Input: part model. Units: mm. Frame: model coordinates. A direction names the side the tool comes from. Round coordinates to 2 decimals unless told otherwise and drop trailing zeros. Loops run counter-clockwise (first coordinate to the right, second up) from the corner with the lowest first, then second, coordinate; pieces in that order, holes last.
(1) Cut plane C-C, the plane z = 80. Output: boundary loops of the cut face in (x, y).
(2) Draft query along Z for faces 3 (the face through (-29, 11, 111.427)), 4 (the face through (-84.149, 12, -41)), 5 (the face through (-27, 11, -194.573)). Return one class per face: released by +Z, released by -Z, zero draft, split by the parting line, or undercut.
(3) Line query: line 1 (X direction, y = 18, z = -43.75); line 2 (X direction, y = 10.75, z = -59.5); line 3 (Z direction, x = -60.5, y = 21.75). Output: solid intervals per line, ascending.
(4) Cut plane B-B, the plane x = -9. Output: boundary loops of the cut face in (y, z), and give its area (3 significant figures).
(5) First-contact query: pin 1 Ø5 at (x, z) = (-52, -162.5) entering from +Y. Flat tip, straight axial feed; report the tip coordinate or a pass-through.
(6) Access query for faces 1 (the face through (-27, -1, -39)), 2 (the face through (-29, 11, 109.927)). Directions: +Z, -Z, +X, -X, +Y, -Y. A direction counts if a zero-diameter tool reaches every point of the face in a straight line with its end or side. Return the directions, or none.
(7) Cut plane A-A, the plane y = 10.25. Output: boundary loops of the cut face in (x, z), and give its area (3 significant figures).
Autodesk Inventor part; units mm, degrees
ref_plane "YZ Plane" through (0, 0, 0) normal (1, 0, 0) x (0, 1, 0)
ref_plane "XZ Plane" through (0, 0, 0) normal (0, 1, 0) x (-1, 0, 0)
ref_plane "XY Plane" through (0, 0, 0) normal (0, 0, 1) x (1, 0, 0)
sketch "Sketch1" plane through (0, 0, 0) normal (0, 1, 0) x (-1, 0, 0)
  line L0 (80.1493, 105.9266) -> (-24.8507, 105.9266) construction
  line L1 (-24.8507, 105.9266) -> (-24.8507, -189.0734) construction
  line L2 (-24.8507, -189.0734) -> (80.1493, -189.0734) construction
  line L3 (80.1493, -189.0734) -> (80.1493, 105.9266) construction
  line L4 (80.1493, 91.9266) -> (83.1493, 91.9266) construction
  line L5 (83.1493, 91.9266) -> (83.1493, 84.3266) construction
  line L6 (83.1493, 84.3266) -> (80.1493, 84.3266) construction
  line L7 (80.1493, 84.3266) -> (80.1493, 91.9266) construction
  point P0 (0, 0)
  dimension "d0" = 295
  dimension "d1" = 105
  dimension "d2" = 7.6
  dimension "d3" = 3
  dimension "d4" = 14
sketch "Sketch2" plane through (0, 0, 0) normal (0, 1, 0) x (-1, 0, 0)
  line L0 (80.1493, -189.0734) -> (80.1493, 105.9266) construction
  line L1 (-24.8507, -189.0734) -> (80.1493, -189.0734) construction
  line L2 (-24.8507, 105.9266) -> (-24.8507, -189.0734) construction
  line L3 (80.1493, 105.9266) -> (-24.8507, 105.9266) construction
  line L4 (90.1493, 109.9266) -> (90.1493, -193.0734)
  line L5 (-34.8507, -193.0734) -> (-34.8507, 109.9266)
  line L6 (90.1493, 109.9266) -> (-34.8507, 109.9266)
  line L7 (90.1493, -193.0734) -> (-34.8507, -193.0734)
  line L8 (91.6493, -194.5734) -> (91.6493, 111.4266)
  line L9 (91.6493, 111.4266) -> (-36.3507, 111.4266)
  line L10 (-36.3507, 111.4266) -> (-36.3507, -194.5734)
  line L11 (-36.3507, -194.5734) -> (91.6493, -194.5734)
  dimension "d71" = 10
  dimension "d72" = 4
  dimension "d73" = 10
  dimension "d74" = 4
  dimension "d75" = 1.5
extrude "Extrusion1" add sketch "Sketch2" against normal blind 1 contours L4 L7 L5 L6
extrude "Extrusion2" add sketch "Sketch2" along normal blind 23 and the other way blind 1
sketch "Sketch5" plane through (-91.6493, -1, 111.4266) normal (-1, 0, 0) x (0, 0, 1)
  circle A0 centre (-246, 6) radius 2.25
  circle A1 centre (-90.8, 6) radius 2.25
  circle A2 centre (-215.2, 6) radius 2.25
  circle A3 centre (-60, 6) radius 2.25
  line L0 (0, 0) -> (0, 24)
  line L1 (-306, 24) -> (0, 24)
  line L2 (-306, 24) -> (-306, 0)
  line L3 (0, 0) -> (-306, 0)
  point P0 (-111.4266, 1)
  dimension "d35" = 4.5
  dimension "d37" = 4.5
  dimension "d39" = 4.5
  dimension "d40" = 0
  dimension "d41" = 30.8
  dimension "d45" = 4.5
  dimension "d46" = 0
  dimension "d47" = 30.8
  dimension "d76" = 60
  dimension "d77" = 60
  dimension "d144" = 18
  dimension "d145" = 18
extrude "Extrusion4" cut sketch "Sketch5" against normal up to surface (1.5 mm away) contours A0 | A1 | A2 | A3
sketch "Sketch7" plane through (-90.1493, 0, -193.0734) normal (1, 0, 0) x (0, 0, -1)
  line L0 (-151.5, 23) -> (-151.5, 0) construction
  line L1 (-141.5, 23) -> (-141.5, 0)
  line L2 (-161.5, 23) -> (-161.5, 0)
  line L3 (-303, 23) -> (0, 23)
  line L4 (-303, 0) -> (0, 0)
  line L5 (0, 23) -> (0, 0)
  dimension "d106" = 10
  dimension "d107" = 10
  dimension "d148" = 151.5
  dimension "d149" = 151.5
extrude "Extrusion6" add sketch "Sketch7" along normal blind 6 contours L1 L4 L2 L3
ref_plane "Work Plane2" through (-27.6493, 0, 109.9266) normal (1, 0, 0) x (0, 0, -1)
ref_plane "Work Plane4" through (-90.1493, 0, -41.5734) normal (0, 0, 1) x (1, 0, 0)
sketch "Sketch16" plane through (-90.1493, 0, -31.5734) normal (0, 0, 1) x (1, 0, 0)
  line L0 (0, 0) -> (0, 23)
  line L1 (0, 23) -> (6, 23)
  point P0 (90.1493, 0)
  point P1 (3.5, 18)
  dimension "d108" = 3.5
  dimension "d109" = 5
hole "Hole3" at (-86.6493, 18, -31.5734) direction (0, 0, -1) diameter 2.6 depth 5 countersink diameter 5 countersink angle 82
sketch "Sketch17" plane through (-86.6493, 18, -36.5734) normal (0, 0, 1) x (1, 0, 0)
  circle A0 centre (0, 0) radius 1.3
  point P0 (86.6493, -18)
hole "Hole4" at (-86.6493, 18, -36.5734) direction (0, 0, -1) diameter 2.6 depth 15 tip angle 118
sketch "Sketch18" plane through (-90.1493, 0, -31.5734) normal (0, 0, 1) x (1, 0, 0)
  line L0 (0, 0) -> (0, 23)
  line L1 (6, 0) -> (0, 0)
  point P0 (90.1493, 0)
  point P1 (3.5, 5)
  point P2 (0, 18)
  dimension "d124" = 3.5
  dimension "d125" = 5
hole "Hole5" at (-86.6493, 5, -31.5734) direction (0, 0, -1) diameter 2.6 depth 5 countersink diameter 5 countersink angle 82
sketch "Sketch19" plane through (-86.6493, 5, -36.5734) normal (0, 0, 1) x (1, 0, 0)
  circle A0 centre (0, 0) radius 1.3
  point P0 (86.6493, -5)
hole "Hole6" at (-86.6493, 5, -36.5734) direction (0, 0, -1) diameter 2.6 depth 15 tip angle 118
mirror "Mirror6" about plane through (-27.6493, 0, 109.9266) normal (1, 0, 0) of "Extrusion6", "Hole3", "Hole5", "Hole4", "Hole6"
sketch "Sketch21" plane through (-90.1493, 0, -41.5734) normal (0, 0, 1) x (1, 0, 0)
  line L0 (-38.4696, 48.4578) -> (185.798, 48.4578)
  line L1 (185.798, 48.4578) -> (185.798, -48.9918)
  line L2 (185.798, -48.9918) -> (-38.4696, -48.9918)
  line L3 (-38.4696, -48.9918) -> (-38.4696, 48.4578)
  point P0 (90.1493, 0)
extrude "Extrusion12" [suppressed]
properties part number "Case Tastiera"
Reported:
1. outline: (-91.65, -1) - (36.35, -1) - (36.35, 23) - (34.85, 23) - (34.85, 0) - (-90.15, 0) - (-90.15, 23) - (-91.65, 23) - close
2. face 3: released by +Z
2. face 4: undercut
2. face 5: released by -Z
3. line 1: x = -91.65 to -87.95, -85.35 to -84.15, 28.85 to 30.05, 32.65 to 36.35
3. line 2: x = -91.65 to -90.15, 34.85 to 36.35
3. line 3: z = -194.57 to -193.07, 109.93 to 111.43
4. outline: (-1, -194.57) - (23, -194.57) - (23, -193.07) - (0, -193.07) - (0, 109.93) - (23, 109.93) - (23, 111.43) - (-1, 111.43) - close
4. area: 375 mm2
5. pin 1: stops at y = 0
6. face 1: +Z, -Z, +X, -X, -Y
6. face 2: +Y
7. outline: (-91.65, -194.57) - (36.35, -194.57) - (36.35, 111.43) - (-91.65, 111.43) - close; hole (-90.15, -193.07) - (34.85, -193.07) - (34.85, -51.57) - (28.85, -51.57) - (28.85, -31.57) - (34.85, -31.57) - (34.85, 109.93) - (-90.15, 109.93) - (-90.15, -31.57) - (-84.15, -31.57) - (-84.15, -51.57) - (-90.15, -51.57) - close
7. area: 1,530 mm2
